The listing builds one solid part. Answer for the finished solid, in the listing's coordinates (mm). Face numbers are marked on the shaded views. A direction names the side the tool comes from. Round coordinates to 2 decimals unless told otherwise and drop trailing zeros. Order: outer loops, then holes, each group sorted by start corner. A loop starts at its lowest first (then second) coordinate and runs counter-clockwise, first axis right, second up. Notation, with made-up numbers: (85.25, -2) - (115.25, -2) arc R27 ccw to (115.25, 18) - close; hole circle Ø5 at (56.25, 81.25). An arc over 180 degrees is marked (long way). One line per item, written item: value. Start each with the question number.
1. Section D-D, the plane x = 6 is taken. Give the vertices of the cut face in (y, z).
2. Section B-B, the plane x = 23.5 is taken. Give the vertices of the cut face in (y, z), then the cut area to 3 significant figures.
3. A tool of negligible diameter and unlimited length cuts with its end or side. For the marked faces 4 and 5, from which of +Z, -Z, +X, -X, +Y, -Y can it reach the whole face along a straight path? Write none if from no direction.
4. Flat-ended cylindrical pins translate along their axes: P1, Ø3, axis at y = 36, z = 97.5, coming from the -X side; P2, Ø2, axis at x = 38, z = 23.5, coming from the +Y side; P3, Ø3, axis at y = 6, z = 68.5, coming from the -X side. Find the tip coordinate at first contact, or state that the pin passes through.
5. Section A-A, the plane y = 26.5 is taken. Give the vertices of the cut face in (x, z).
6. For a pull along Z with two mould halves and no side action, classify the marked faces 1, 2 and 3 as released by +Z, released by -Z, zero draft, split by the parting line, or undercut.
7. Straight lines are drawn through the part: line 1 (Z direction, x = 95, y = 39); line 2 (Z direction, x = 86.5, y = 65); line 3 (Y direction, x = 92.5, z = 50). For each, find the intervals that lie inside material, in ascending order.
8. Section C-C, the plane y = 49.5 is taken. Give the vertices of the cut face in (x, z).
from build123d import *

# Parameters (mm, degrees)
F1_DEPTH = 10
F3_DEPTH = 10
F5_DEPTH = 10
F6_W     = 9.066966
F6_H     = 10
F7_DEPTH = 80


with BuildPart() as f1:
    # F0 (on Front) → F1 (new body)
    with BuildSketch(Plane.XZ):
        Polygon((0, 100), (0, 0), (18.133933, 0), (18.133933, 33.002501), (81.866067, 0), (100, 0), (100, 18.133933), (38.462467, 50), (100, 81.866067), (100, 100), (81.866067, 100), (18.133933, 66.997499), (18.133933, 100), align=None)
    extrude(amount=F1_DEPTH)

    # F2 (on face) → F3 (join)
    with BuildSketch(Plane.YZ.offset(100)):
        with BuildLine():
            Line((60.558972, 77.197799), (70, 88.853999))
            ThreePointArc((70, 88.853999), (55.222721, 97.1312), (38.529907, 100))
            ThreePointArc((38.529907, 100), (-11.470093, 50), (38.529907, 0))
            ThreePointArc((38.529907, 0), (55.222721, 2.8688), (70, 11.146001))
            Line((70, 11.146001), (60.558972, 22.802201))
            ThreePointArc((60.558972, 22.802201), (3.529907, 50), (60.558972, 77.197799))
        make_face()
    extrude(amount=-F3_DEPTH)

    # F4 (on face) → F5 (join)
    with BuildSketch(Plane.XY.offset(100)):
        Polygon((0, -10), (18.133933, -10), (18.133933, 55), (50, 13.471332), (81.866067, 55), (81.866067, -10), (100, -10), (100, 80), (81.866067, 80), (50, 38.471332), (18.133933, 80), (0, 80), align=None)
    extrude(amount=-F5_DEPTH)

    # F6 (on face) → F7 (join)
    with BuildSketch(Plane(origin=(0, 0, 0), x_dir=(-1, 0, 0), z_dir=(0, 1, 0))):
        with Locations((-4.533483, 5)):
            Rectangle(F6_W, F6_H)
    extrude(amount=F7_DEPTH)


solid = f1.part
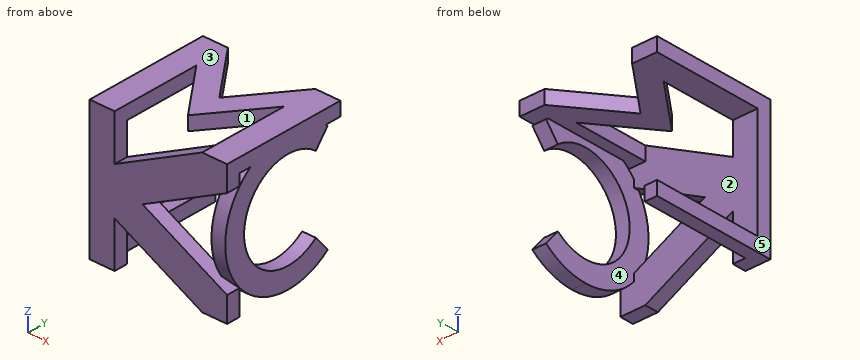
Answer list:
1. outline: (-10, 0) - (80, 0) - (80, 10) - (0, 10) - (0, 90) - (80, 90) - (80, 100) - (-10, 100) - close
2. outline: (-10, 30.22) - (0, 30.22) - (0, 69.78) - (-10, 69.78) - close; (48.01, 90) - (73.01, 90) - (73.01, 100) - (48.01, 100) - close
2. area: 646 mm²
3. face 4: +Y
3. face 5: +Z, -Z, -X, +Y, -Y
4. P1: stops at x = 0
4. P2: stops at y = 0
4. P3: stops at x = 90
5. outline: (0, 0) - (9.07, 0) - (9.07, 10) - (0, 10) - close; (0, 90) - (18.13, 90) - (18.13, 100) - (0, 100) - close; (40, 90) - (60, 90) - (60, 100) - (40, 100) - close; (81.87, 90) - (90, 90) - (90, 82.87) - (100, 82.87) - (100, 100) - (81.87, 100) - close; (90, 1.47) - (100, 1.47) - (100, 17.13) - (90, 17.13) - close
6. face 1: zero draft
6. face 2: undercut
6. face 3: released by +Z
7. line 1: z = 0 to 15, 85 to 100
7. line 2: z = 90 to 100
7. line 3: y = -11.47 to 3.53
8. outline: (0, 0) - (9.07, 0) - (9.07, 10) - (0, 10) - close; (0, 90) - (18.13, 90) - (18.13, 100) - (0, 100) - close; (22.35, 90) - (41.54, 90) - (41.54, 100) - (22.35, 100) - close; (58.46, 90) - (77.65, 90) - (77.65, 100) - (58.46, 100) - close; (81.87, 90) - (90, 90) - (90, 83.24) - (100, 83.24) - (100, 100) - (81.87, 100) - close; (90, 1.22) - (100, 1.22) - (100, 16.76) - (90, 16.76) - close
